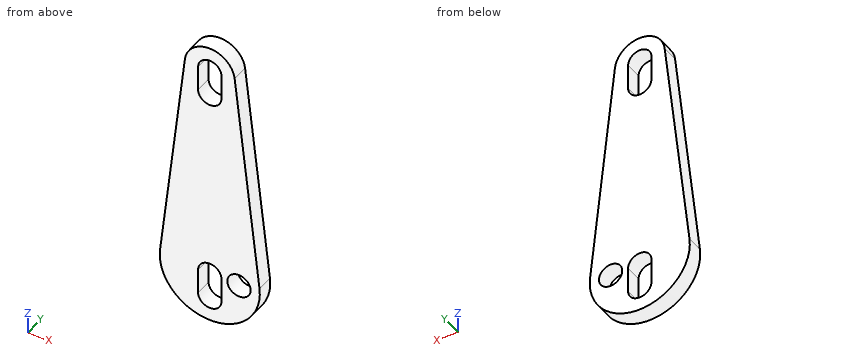
```python
from build123d import *

# Parameters (mm, degrees)
SKETCH1_R           = 1.4
BOSS_EXTRUDE1_DEPTH = 2


with BuildPart() as part:
    # Sketch1 → Boss-Extrude1 (new body)
    with BuildSketch(Plane(origin=(0, 0, 0), x_dir=(1, 0, 0), z_dir=(0, 1, 0))):
        with BuildLine():
            Line((-5.961660753, 25.902799097), (-2.980830377, -0.338600451))
            ThreePointArc((-2.980830377, -0.338600451), (0, -3), (2.980830377, -0.338600451))
            Line((2.980830377, -0.338600451), (5.961660753, 25.902799097))
            ThreePointArc((5.961660753, 25.902799097), (0, 32.58), (-5.961660753, 25.902799097))
        make_face()
        with Locations((3.5, 26.58)):
            Circle(SKETCH1_R, mode=Mode.SUBTRACT)
        with BuildLine():
            Line((-1.4, 0), (-1.4, 3))
            ThreePointArc((-1.4, 3), (0, 4.4), (1.4, 3))
            Line((1.4, 3), (1.4, 0))
            ThreePointArc((1.4, 0), (0, -1.4), (-1.4, 0))
        make_face(mode=Mode.SUBTRACT)
        with BuildLine():
            Line((1.4, 29.59), (1.4, 26.59))
            ThreePointArc((1.4, 26.59), (0, 25.19), (-1.4, 26.59))
            Line((-1.4, 26.59), (-1.4, 29.59))
            ThreePointArc((-1.4, 29.59), (0, 30.99), (1.4, 29.59))
        make_face(mode=Mode.SUBTRACT)
    extrude(amount=BOSS_EXTRUDE1_DEPTH)


solid = part.part
```
Work out the finished part from the listing and answer in its coordinate system (mm). Coordinates: 2 decimals unless noted, no trailing zeros. Loops run counter-clockwise (first coordinate to the right, second up) from the corner with the lowest first, then second, coordinate; pieces in that order, holes last. Notation, with made-up numbers: (6.25, 19) - (62.25, 19) arc R30 ccw to (62.25, 44) - close; hole circle Ø6 at (88, -4.5). An arc over 180 degrees is marked (long way). Use a Markdown table: item, result.
Item 1: Find section B-B, the plane y = 0.65. Determine the outline of the cut face in (x, z).
Evaluation:
| item | result |
|---|---|
| outline | (-5.96, -25.9) arc R6 ccw (long way) to (5.96, -25.9) - (2.98, 0.34) arc R3 ccw to (-2.98, 0.34) - close; hole (-1.4, -29.59) arc R1.4 ccw to (1.4, -29.59) - (1.4, -26.59) arc R1.4 ccw to (-1.4, -26.59) - close; hole (-1.4, -3) arc R1.4 ccw to (1.4, -3) - (1.4, 0) arc R1.4 ccw to (-1.4, 0) - close; hole circle Ø2.8 at (3.5, -26.58) |
Item 2: Find section C-C, the plane x = 4.5. Determine the outline of the cut face in (y, z).
Evaluation:
| item | result |
|---|---|
| outline | (0, -30.55) - (2, -30.55) - (2, -27.56) - (0, -27.56) - close; (0, -25.6) - (2, -25.6) - (2, -13.04) - (0, -13.04) - close |
Item 3: Find section A-A, the plane x = -1. Determine the outline of the cut face in (y, z).
Evaluation:
| item | result |
|---|---|
| outline | (0, -32.5) - (2, -32.5) - (2, -30.57) - (0, -30.57) - close; (0, -25.61) - (2, -25.61) - (2, -3.98) - (0, -3.98) - close; (0, 0.98) - (2, 0.98) - (2, 2.83) - (0, 2.83) - close |
Item 4: Given pin 1 Ø0.6 at (y, z) = (1, -1.5) entering from -X; pin 2 Ø0.6 at (y, z) = (1, -28) entering from -X; pin 3 Ø0.6 at (y, z) = (0.5, -2) entering from +X, each flat-ended and moving along its own axis, determine where each tip first touches the part or whether it passes through.
Evaluation:
| item | result |
|---|---|
| pin 1 | stops at x = -3.22 |
| pin 2 | stops at x = -5.89 |
| pin 3 | stops at x = 3.28 |
Item 5: Find section D-D, the plane x = 2.5. Determine the outline of the cut face in (y, z), and give its area (3 significant figures).
Evaluation:
| item | result |
|---|---|
| outline | (0, -32.03) - (2, -32.03) - (2, -27.56) - (0, -27.56) - close; (0, -25.6) - (2, -25.6) - (2, 1.66) - (0, 1.66) - close |
| area | 63.5 mm2 |
Item 6: Consider probe 1 along X at (y, z) = (0.8, -26.58); probe 2 along Z at (x, y) = (1, 0.9); probe 3 along X at (y, z) = (1.1, 1). Determine where each line is inside the solid, lowest interval first. Write a range as from..to.
Evaluation:
| item | result |
|---|---|
| probe 1 | x = -6..-1.4, 1.4..2.1, 4.9..6 |
| probe 2 | z = -32.5..-30.57, -25.61..-3.98, 0.98..2.83 |
| probe 3 | x = -2.83..-0.98, 0.98..2.83 |
